Could you check a few things on this model? Use its own coordinates, in mm. Coordinates: 2 decimals unless noted, no trailing zeros. Loops run counter-clockwise (first coordinate to the right, second up) from the corner with the lowest first, then second, coordinate; pieces in that order, holes last. Notation, with made-up numbers: M -19,12 L -11,12 A12 cw -11,28 Z; hole C -23.75,87 d3. An arc over 180 degrees is marked long. Write each question's results on one line, items separated by ' | '.
Autodesk Inventor part; units mm, degrees
ref_plane "YZ Plane" through (0, 0, 0) normal (1, 0, 0) x (0, 1, 0)
ref_plane "XZ Plane" through (0, 0, 0) normal (0, 1, 0) x (-1, 0, 0)
ref_plane "XY Plane" through (0, 0, 0) normal (0, 0, 1) x (1, 0, 0)
sketch "Sketch1" plane through (0, 0, 0) normal (0, 1, 0) x (-1, 0, 0)
  circle A0 centre (0, 0) radius 21.082
  circle A1 centre (0, 0) radius 17.526
  dimension "d0" = 42.164
  dimension "d1" = 35.052
extrude "Extrusion1" add sketch "Sketch1" along normal mid plane 469.1126
sketch "Sketch2" plane through (0, 0, 0) normal (0, 0, 1) x (1, 0, 0)
  circle A0 centre (0, 245.7006) radius 21.082
  line L0 (21.082, 234.5563) -> (-21.082, 234.5563)
  line L1 (-21.082, -234.5563) -> (21.082, -234.5563)
  line L2 (-21.082, -234.5563) -> (-21.082, 234.5563)
  arc A1 (-21.082, -231.3813) -> (-17.907, -234.5563) centre (-17.907, -231.3813) ccw
  point P0 (0, 0)
  dimension "d4" = 42.164
  dimension "d6" = 11.1442
  dimension "d7" = 6.35
extrude "Extrusion2" cut sketch "Sketch2" against normal through all both and the other way through all
properties part number "FE-110-002 Upright Middle Section" material "Aluminum 6061"
(1) Imagine slicing it at B-B, the plane z = 0. List the corners of the cut face in (x, y) for me (3 decimals).
Reported:
outline: M -21.082,-231.381 A3.175 ccw -17.907,-234.556 L -17.526,-234.556 L -17.526,233.984 A21.082 cw -17.896,234.556 L -21.082,234.556 Z; M 17.526,-234.556 L 21.082,-234.556 L 21.082,234.556 L 17.896,234.556 A21.082 cw 17.526,233.984 Z
(2) Will these pins go through, and if not, where does the flat tip stop? P1, Ø1.5, axis at y = 120.5, z = -8.5, coming from the -X side; P2, Ø3, axis at x = -17, y = -168, coming from the -Z side; P3, Ø5, axis at y = 159.5, z = 11, coming from the -X side.
Reported:
P1: stops at x = -19.61 | P2: stops at z = -14.29 | P3: stops at x = -19.29
(3) Please list where these lines run through material, in increasing order: probe 1 along X at (y, z) = (-24, 0); probe 2 along X at (y, z) = (-85.5, -11). Write a range as from..to.
Reported:
probe 1: x = -21.08..-17.53, 17.53..21.08 | probe 2: x = -17.98..-13.64, 13.64..17.98
(4) If we mould it in two halves opening along X, with no side actions, what happens to faces 1 (the flat face through (18, -234.556, -1)), 2 (the cylindrical face through (-20.11, -3.28, -6.33)), 3 (the cylindrical face through (-16.72, -3.57, -5.26)), 4 (the cylindrical face through (-14.46, 230.36, -10.83))? For each: released by +X, released by -X, zero draft, split by the parting line, or undercut.
Reported:
face 1: zero draft | face 2: split by the parting line | face 3: undercut | face 4: undercut
(5) Imagine slicing it at C-C, the plane y = 79. List the corners of the cut face in (x, z) for me, and give its area (3 significant figures).
Reported:
outline: C 0,0 d42.16; hole C 0,0 d35.05 | area: 431 mm2
(6) Imagine slicing it at A-A, the plane x = 0. List the corners of the cut face in (y, z) for me.
Reported:
outline: M -234.56,-21.08 L 224.62,-21.08 L 224.62,-17.53 L -234.56,-17.53 Z; M -234.56,17.53 L 224.62,17.53 L 224.62,21.08 L -234.56,21.08 Z
